```python
from build123d import *

# Parameters (mm, degrees)
SKETCH1_W           = 40
SKETCH1_H           = 40
BOSS_EXTRUDE1_DEPTH = 8.5
FILLET1_R           = 10
CUT_EXTRUDE1_DEPTH  = 3
SKETCH4_R           = 5
CUT_EXTRUDE2_DEPTH  = 29.814059068
SKETCH5_R           = 1.6
CUT_EXTRUDE3_DEPTH  = 30.533878851
CUT_EXTRUDE4_DEPTH  = 3
SKETCH8_R           = 12.5
CUT_EXTRUDE5_DEPTH  = 1.5


with BuildPart() as part:
    # Sketch1 → Boss-Extrude1 (new body)
    with BuildSketch(Plane(origin=(0, 0, 0), x_dir=(0, 0, -1), z_dir=(1, 0, 0))):
        Rectangle(SKETCH1_W, SKETCH1_H)
    extrude(amount=BOSS_EXTRUDE1_DEPTH)

    # Fillet1
    fillet1_edges = [part.edges().sort_by_distance(p)[0] for p in [
        (4.25, -20, -20),
        (4.25, -20, 20),
        (4.25, 20, 20),
        (4.25, 20, -20),
    ]]
    fillet(fillet1_edges, radius=FILLET1_R)

    # Sketch2 → Cut-Extrude1 (cut)
    with BuildSketch(Plane(origin=(8.5, 0, 0), x_dir=(0, 0, -1), z_dir=(1, 0, 0))):
        Polygon((-1.944543648, -13.258252147), (13.258252147, 1.944543648), (1.944543648, 13.258252147), (-13.258252147, -1.944543648), align=None)
    extrude(amount=-CUT_EXTRUDE1_DEPTH, mode=Mode.SUBTRACT)

    # Sketch4 → Cut-Extrude2 (cut, through all)
    with BuildSketch(Plane(origin=(5.5, 0, 0), x_dir=(0, 0, -1), z_dir=(1, 0, 0))):
        Circle(SKETCH4_R)
    extrude(amount=-CUT_EXTRUDE2_DEPTH, mode=Mode.SUBTRACT)

    # Sketch5 → Cut-Extrude3 (cut, through all)
    with BuildSketch(Plane(origin=(8.5, 0, 0), x_dir=(0, 0, -1), z_dir=(1, 0, 0))):
        with Locations((-12.5, 12.5)):
            Circle(SKETCH5_R)
        with Locations((-12.5, -12.5)):
            Circle(SKETCH5_R)
        with Locations((12.5, -12.5)):
            Circle(SKETCH5_R)
        with Locations((12.5, 12.5)):
            Circle(SKETCH5_R)
    extrude(amount=-CUT_EXTRUDE3_DEPTH, mode=Mode.SUBTRACT)

    # Sketch7 → Cut-Extrude4 (cut)
    with BuildSketch(Plane(origin=(8.5, 0, 0), x_dir=(0, 0, -1), z_dir=(1, 0, 0))):
        Polygon((14.142135624, -21.213203436), (-21.213203436, 14.142135624), (-14.142135624, 21.213203436), (21.213203436, -14.142135624), align=None)
    extrude(amount=-CUT_EXTRUDE4_DEPTH, mode=Mode.SUBTRACT)

    # Sketch8 → Cut-Extrude5 (cut)
    with BuildSketch(Plane.ZY):
        Circle(SKETCH8_R)
    extrude(amount=-CUT_EXTRUDE5_DEPTH, mode=Mode.SUBTRACT)


solid = part.part
```
Design review of the part built by this model. Coordinates are the model's own, in mm. A direction names the side the tool comes from. Coordinates: 2 decimals unless noted, no trailing zeros. Order: outer loops, then holes, each group sorted by start corner. A loop starts at its lowest first (then second) coordinate and runs counter-clockwise, first axis right, second up. Notation, with made-up numbers: M 42.25,-33 L 52.25,-33 A10 ccw 52.25,-19 Z; hole C -33.75,-23.75 d5. An arc over 180 degrees is marked long. Answer as a JSON object with one key per item and string values. Group by question number.
1) Add section B-B, the plane y = 4.5. Write out the cut boundary in (x, z).
2) Mouldability with a two-part tool opening along Y and no side actions: class faces 4 (the cylindrical face through (2.79, 12.57, 14.1)), 5 (the flat face through (4, 0, 20)), 6 (the flat face through (4, -20, 0)) as pulls with the +Y half, pulls with the -Y half, needs draft (parallel to the pull), parting line crosses it, or undercut.
3) Wall thickness on L1, parallel to Y at x = 3.45, z = 12.5; L2, parallel to Y at x = 1.1, z = 0; L3, parallel to X at y = 4, z = -5: over which ranges is each line inside the solid? List them lowest first.
4) For pin 1 (3.5 mm diameter, centred on y = -12.5, z = -12.5, fed in from +X); pin 2 (11.5 mm diameter, centred on y = 0, z = 0, fed in from -X); pin 3 (3 mm diameter, centred on y = 12.5, z = -12.5, fed in from +X), all flat-tipped, find the tip position at first contact; note any pin that passes through.
5) Tool access review of faces 1 (the flat face through (7.02, 7.28, 14.35)), 2 (the flat face through (1.5, -5.4, -0.2)), 3 (the cylindrical face through (3.53, -4.88, 1.08)): name each direction out of +Z, -Z, +X, -X, +Y, -Y from which nothing blocks a thin tool from reaching the whole face with its end or side.
6) Add section A-A, the plane x = 7.75. Write out the cut boundary in (y, z), then the cut area to 3 significant figures.
7) Add section C-C, the plane z = 0. Write out the cut boundary in (x, y).
8) Add section D-D, the plane x = 2.25. Write out the cut boundary in (y, z), then the cut area to 3 significant figures.
Computed values:
{
 "1": {"outline": "M 0,-20 L 8.5,-20 L 8.5,-10.7 L 5.5,-10.7 L 5.5,-2.18 L 1.5,-2.18 L 1.5,-11.66 L 0,-11.66 Z; M 0,11.66 L 1.5,11.66 L 1.5,2.18 L 5.5,2.18 L 5.5,11.57 L 8.5,11.57 L 8.5,20 L 0,20 Z"},
 "2": {"face 4": "undercut", "face 5": "needs draft", "face 6": "pulls with the -Y half"},
 "3": {"L1": "y = -19.68 to -14.1, -10.9 to 10.9, 14.1 to 19.68", "L2": "y = -20 to -12.5, 12.5 to 20", "L3": "x = 1.5 to 5.5"},
 "4": {"pin 1": "stops at x = 5.5", "pin 2": "stops at x = 1.5", "pin 3": "passes through"},
 "5": {"face 1": "+X", "face 2": "-X", "face 3": "+X, -X"},
 "6": {"outline": "M -20,-10 A10 ccw -19.66,-12.59 L -9.19,-2.12 L -13.26,1.94 L -1.94,13.26 L 2.12,9.19 L 12.59,19.66 A10 ccw 10,20 L -10,20 A10 ccw -20,10 Z; M -12.59,-19.66 A10 ccw -10,-20 L 10,-20 A10 ccw 20,-10 L 20,10 A10 ccw 19.66,12.59 L 9.19,2.12 L 13.26,-1.94 L 1.94,-13.26 L -2.12,-9.19 Z; hole C -12.5,12.5 d3.2; hole C 12.5,-12.5 d3.2", "area": "840 mm^2"},
 "7": {"outline": "M 0,-20 L 8.5,-20 L 8.5,-11.31 L 5.5,-11.31 L 5.5,-5 L 1.5,-5 L 1.5,-12.5 L 0,-12.5 Z; M 0,12.5 L 1.5,12.5 L 1.5,5 L 5.5,5 L 5.5,11.31 L 8.5,11.31 L 8.5,20 L 0,20 Z"},
 "8": {"outline": "M -20,-10 A10 ccw -10,-20 L 10,-20 A10 ccw 20,-10 L 20,10 A10 ccw 10,20 L -10,20 A10 ccw -20,10 Z; hole C -12.5,-12.5 d3.2; hole C -12.5,12.5 d3.2; hole C 0,0 d10; hole C 12.5,-12.5 d3.2; hole C 12.5,12.5 d3.2", "area": "1,400 mm^2"}
}
